CAD build for the part. Positions are in the model's coordinates, mm. Face numbers are marked on the shaded views. A direction names the side the tool comes from. Give positions to 0.01 mm unless a question says otherwise; leave off trailing zeros. Write each loop counter-clockwise with the first axis right and the second up, starting at its lowest first coordinate (ties: lowest second). Pieces come first, ordered by that corner, then holes. Notation, with made-up numbers: (-13.75, 23.5) -> (40.25, 23.5) arc R16 cw to (40.25, 37.5) -> close; hole circle Ø3 at (20, 69.25). An arc over 180 degrees is marked (long way). Answer in a Markdown table with one row per item. Add a question column.
```python
from build123d import *

# Parameters (mm, degrees)
SKETCH1_W           = 180
SKETCH1_H           = 30
BOSS_EXTRUDE1_DEPTH = 50
CUT_EXTRUDE1_DEPTH  = 108.238052948
CUT_EXTRUDE2_DEPTH  = 108.238052948
SKETCH4_W           = 8
SKETCH4_H           = 30
BOSS_EXTRUDE2_DEPTH = 25
SKETCH5_W           = 7
SKETCH5_H           = 5
BOSS_EXTRUDE3_DEPTH = 7
CUT_EXTRUDE3_DEPTH  = 101.444014257
SKETCH7_R           = 2
CUT_EXTRUDE4_DEPTH  = 15
SKETCH8_R           = 2
CUT_EXTRUDE5_DEPTH  = 110.652369188


with BuildPart() as part:
    # Sketch1 → Boss-Extrude1 (new body)
    with BuildSketch(Plane.XY):
        Rectangle(SKETCH1_W, SKETCH1_H)
    extrude(amount=BOSS_EXTRUDE1_DEPTH)

    # Sketch2 → Cut-Extrude1 (cut, through all)
    with BuildSketch(Plane.XZ.offset(15)):
        Polygon((-90, 9.270509831), (-61.468304511, 0), (-90, 0), align=None)
    extrude(amount=-CUT_EXTRUDE1_DEPTH, mode=Mode.SUBTRACT)

    # Sketch3 → Cut-Extrude2 (cut, through all)
    with BuildSketch(Plane.XZ.offset(15)):
        Polygon((-90, 17.682207625), (-60.201228989, 8), (90, 8), (90, 50), (-90, 50), align=None)
    extrude(amount=-CUT_EXTRUDE2_DEPTH, mode=Mode.SUBTRACT)

    # Sketch4 → Boss-Extrude2 (add)
    with BuildSketch(Plane.XY.offset(8)):
        with Locations((86, 0)):
            Rectangle(SKETCH4_W, SKETCH4_H)
    extrude(amount=BOSS_EXTRUDE2_DEPTH)

    # Sketch5 → Boss-Extrude3 (add)
    with BuildSketch(Plane.ZY.offset(-82)):
        with Locations((11.5, -12.5)):
            Rectangle(SKETCH5_W, SKETCH5_H)
        with Locations((11.5, 12.5)):
            Rectangle(SKETCH5_W, SKETCH5_H)
    extrude(amount=BOSS_EXTRUDE3_DEPTH)

    # Sketch6 → Cut-Extrude3 (cut, through all)
    with BuildSketch(Plane.XZ.offset(15)):
        Polygon((75, 8), (82, 15), (75, 15), align=None)
    extrude(amount=-CUT_EXTRUDE3_DEPTH, mode=Mode.SUBTRACT)

    # Sketch7 → Cut-Extrude4 (cut)
    with BuildSketch(Plane.ZY.offset(-82)):
        with Locations((20.5, 0)):
            Circle(SKETCH7_R)
    extrude(amount=-CUT_EXTRUDE4_DEPTH, mode=Mode.SUBTRACT)

    # Sketch8 → Cut-Extrude5 (cut, through all)
    with BuildSketch(Plane(origin=(-5.869700773, 0, -18.065081438), x_dir=(-0.9510565162951532, 0, 0.30901699437494884), z_dir=(-0.30901699437494884, 0, -0.9510565162951532))):
        with Locations((74.92439222, 7.5)):
            Circle(SKETCH8_R)
        with Locations((74.92439222, -7.5)):
            Circle(SKETCH8_R)
    extrude(amount=-CUT_EXTRUDE5_DEPTH, mode=Mode.SUBTRACT)


solid = part.part
```
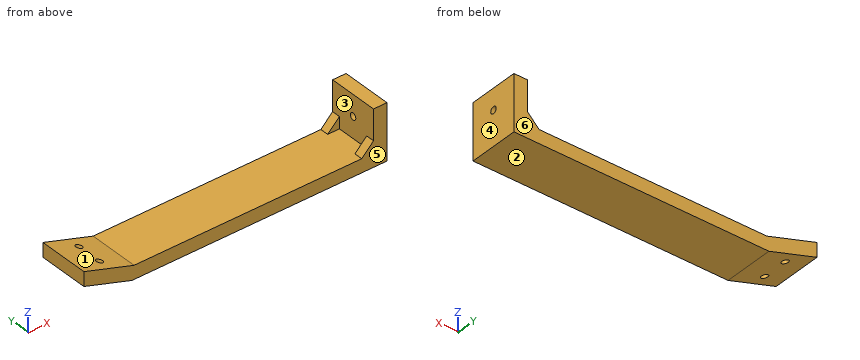
Item 1: Slice it at C-C, the plane y = -12. List the corners of the cut face in (x, z), then the cut area to 3 significant figures.
Item 2: Mould opens along Y. For the marked faces 3, 4, 5 and 6 say: released by +Y, released by -Y, zero draft, split by the parting line, or undercut.
Item 3: Drop flat-ended pins along their axis: pin 1 Ø1.5 at (y, z) = (-5.5, 22) entering from -X; pin 2 Ø3.5 at (x, z) = (77, 11) entering from +Y; pin 3 Ø9 at (x, y) = (-8, -1) entering from +Z. Give the stop position or say it passes through.
Item 4: Probe L1, parallel to Y at x = 86.5, z = 20.5; L2, parallel to X at y = -13.5, z = 31.5; L3, parallel to Z at x = 70, y = 7.5. List the from-to ranges inside material, lowest first. Write a range as from..to.
Item 5: Slice it at D-D, the plane x = -33.5. List the corners of the cut face in (y, z).
Item 6: Slice it at A-A, the plane z = 20.5. List the corners of the cut face in (x, y).
Item 7: Which spindle directions (+Z, -Z, +X, -X, +Y, -Y) get a long thin tool onto all of the face, cutting with end or side? Do the marked faces 1 and 2. Say none if no direction does.
Item 8: Slice it at B-B, the plane y = 0. List the corners of the cut face in (x, z).
Answer key:
| question | item | result |
|---|---|---|
| 1 | outline | (-90, 9.27) -> (-61.47, 0) -> (90, 0) -> (90, 33) -> (82, 33) -> (82, 15) -> (75, 8) -> (-60.2, 8) -> (-90, 17.68) -> close |
| 1 | area | 1,680 mm² |
| 2 | face 3 | undercut |
| 2 | face 4 | zero draft |
| 2 | face 5 | released by -Y |
| 2 | face 6 | released by +Y |
| 3 | pin 1 | stops at x = 82 |
| 3 | pin 2 | stops at y = 15 |
| 3 | pin 3 | stops at z = 8 |
| 4 | L1 | y = -15..-2, 2..15 |
| 4 | L2 | x = 82..90 |
| 4 | L3 | z = 0..8 |
| 5 | outline | (-15, 0) -> (15, 0) -> (15, 8) -> (-15, 8) -> close |
| 6 | outline | (82, -15) -> (90, -15) -> (90, -2) -> (82, -2) -> close; (82, 2) -> (90, 2) -> (90, 15) -> (82, 15) -> close |
| 7 | face 1 | +Z, +Y, -Y |
| 7 | face 2 | -Z, +X, -X, +Y, -Y |
| 8 | outline | (-90, 9.27) -> (-61.47, 0) -> (90, 0) -> (90, 18.5) -> (82, 18.5) -> (82, 8) -> (-60.2, 8) -> (-90, 17.68) -> close; (82, 22.5) -> (90, 22.5) -> (90, 33) -> (82, 33) -> close |
